Design review of the part built by this model. Coordinates are the model's own, in mm. A direction names the side the tool comes from. Give positions to 0.01 mm unless a question says otherwise; leave off trailing zeros. Order: outer loops, then holes, each group sorted by start corner. A loop starts at its lowest first (then second) coordinate and runs counter-clockwise, first axis right, second up. Notation, with made-up numbers: M 6.5,24.25 L 17.5,24.25 A12 ccw 17.5,35.25 Z; hole C 20,10.25 d11. An arc over 180 degrees is marked long. Answer as a JSON object with one key per item and string values.
from build123d import *

# Parameters (mm, degrees)
F0_W      = 31.8
F0_H      = 15.8
F1_DEPTH  = 4.8
F2_W      = 29.4
F2_H      = 13.4
F3_DEPTH  = 8.4
F4_R      = 2.409
F5_DEPTH  = 1.8
F6_R      = 1.3
F7_DEPTH  = 1.2
F8_R      = 2.409
F9_DEPTH  = 8.4
F10_W     = 0.3
F10_H     = 0.6
F11_DEPTH = 8.4
F12_W     = 0.6
F12_H     = 0.3
F13_DEPTH = 8.4
F14_W     = 0.8
F14_H     = 3.4696710694
F15_DEPTH = 6.4


with BuildPart() as f1:
    # F0 (on Top) → F1 (new body, symmetric)
    with BuildSketch(Plane.XY):
        Rectangle(F0_W, F0_H)
    extrude(amount=F1_DEPTH, both=True)

    # F2 (on face) → F3 (cut)
    with BuildSketch(Plane(origin=(0, 0, -4.8), x_dir=(1, 0, 0), z_dir=(0, 0, -1))):
        Rectangle(F2_W, F2_H)
    extrude(amount=-F3_DEPTH, mode=Mode.SUBTRACT)

    # F4 (on face) → F5 (join)
    with BuildSketch(Plane.XY.offset(4.8)):
        with Locations((-12.291, 4.2910612803)):
            Circle(F4_R)
        with Locations((12.291, 4.2910612803)):
            Circle(F4_R)
        with Locations((-12.291, -4.2910612803)):
            Circle(F4_R)
        with Locations((12.291, -4.2910612803)):
            Circle(F4_R)
        with Locations((-4.291, 4.2910612803)):
            Circle(F4_R)
        with Locations((4.291, 4.2910612803)):
            Circle(F4_R)
        with Locations((-4.291, -4.2910612803)):
            Circle(F4_R)
        with Locations((4.291, -4.2910612803)):
            Circle(F4_R)
    extrude(amount=F5_DEPTH)

    # F6 (on face) → F7 (cut)
    with BuildSketch(Plane(origin=(0, 0, 3.6), x_dir=(1, 0, 0), z_dir=(0, 0, -1))):
        with Locations((-11.8301756735, 4)):
            Circle(F6_R)
        with Locations((-3.8301756735, 5.6396185296)):
            Circle(F6_R)
        with Locations((4, 4)):
            Circle(F6_R)
        with Locations((12, 4)):
            Circle(F6_R)
        with Locations((-11.8301756735, -4)):
            Circle(F6_R)
        with Locations((-3.8301756735, -5.6396185296)):
            Circle(F6_R)
        with Locations((4, -4)):
            Circle(F6_R)
        with Locations((12, -4)):
            Circle(F6_R)
    extrude(amount=-F7_DEPTH, mode=Mode.SUBTRACT)

    # F8 (on face) → F9 (join, through all)
    with BuildSketch(Plane(origin=(0, 0, 3.6), x_dir=(1, 0, 0), z_dir=(0, 0, -1))):
        Circle(F8_R)
    extrude(amount=F9_DEPTH)

    # F10 (on face) → F11 (join, through all)
    with BuildSketch(Plane(origin=(0, 0, 3.6), x_dir=(1, 0, 0), z_dir=(0, 0, -1))):
        with Locations((-14.55, 4)):
            Rectangle(F10_W, F10_H)
        with Locations((-14.55, -4)):
            Rectangle(F10_W, F10_H)
        with Locations((14.55, 4)):
            Rectangle(F10_W, F10_H)
        with Locations((14.55, -4)):
            Rectangle(F10_W, F10_H)
    extrude(amount=F11_DEPTH)

    # F12 (on face) → F13 (join, through all)
    with BuildSketch(Plane(origin=(0, 0, 3.6), x_dir=(1, 0, 0), z_dir=(0, 0, -1))):
        with Locations((-11.8301756735, 6.55)):
            Rectangle(F12_W, F12_H)
        with Locations((-3.8301756735, 6.55)):
            Rectangle(F12_W, F12_H)
        with Locations((4, 6.55)):
            Rectangle(F12_W, F12_H)
        with Locations((12.3396486531, 6.55)):
            Rectangle(F12_W, F12_H)
        with Locations((-3.8301756735, -6.55)):
            Rectangle(F12_W, F12_H)
        with Locations((-11.8301756735, -6.55)):
            Rectangle(F12_W, F12_H)
        with Locations((4, -6.55)):
            Rectangle(F12_W, F12_H)
        with Locations((12.3396486531, -6.55)):
            Rectangle(F12_W, F12_H)
    extrude(amount=F13_DEPTH)

    # F14 (on face) → F15 (join)
    with BuildSketch(Plane(origin=(0, 0, 3.6), x_dir=(1, 0, 0), z_dir=(0, 0, -1))):
        with Locations((0, 4.9651644653)):
            Rectangle(F14_W, F14_H)
        with Locations((0, -4.9651644653)):
            Rectangle(F14_W, F14_H)
    extrude(amount=F15_DEPTH)


solid = f1.part
(1) We need section B-B (z = -0.5). Count the separate pieces of the cut face and the enclosed holes in it, plus the area to 3 significant figures.
Checked values:
{"separate pieces": "2", "enclosed holes": "1", "area": "134 mm^2"}
(2) We need section D-D (z = 5.25). Write out the cut boundary in (x, y), plus the area to 3 significant figures.
Checked values:
{"outline": "C -12.29,-4.29 d4.82; C -12.29,4.29 d4.82; C -4.29,-4.29 d4.82; C -4.29,4.29 d4.82; C 4.29,-4.29 d4.82; C 4.29,4.29 d4.82; C 12.29,-4.29 d4.82; C 12.29,4.29 d4.82", "area": "146 mm^2"}
(3) To check wall thickness, follow L1, parallel to X at y = 3.75, z = -1.75; L2, parallel to Y at x = 12, z = 4.55; L3, parallel to X at y = 4, z = 4.5. State the ranges of each line that lie inside material, in increasing order. Write a range as from..to.
Checked values:
{"L1": "x = -15.9..-14.4, -0.4..0.4, 14.4..15.9", "L2": "y = -7.9..-5.3, -2.7..2.7, 5.3..7.9", "L3": "x = -15.9..-13.13, -10.53..2.7, 5.3..10.7, 13.3..15.9"}
(4) We need section A-A (x = 7.5). Write out the cut boundary in (y, z).
Checked values:
{"outline": "M -7.9,-4.8 L -6.7,-4.8 L -6.7,3.6 L 6.7,3.6 L 6.7,-4.8 L 7.9,-4.8 L 7.9,4.8 L -7.9,4.8 Z"}
(5) We need section C-C (y = -1.5). Write out the cut boundary in (x, z), plus the area to 3 significant figures.
Checked values:
{"outline": "M -15.9,-4.8 L -14.7,-4.8 L -14.7,3.6 L -1.89,3.6 L -1.89,-4.8 L 1.89,-4.8 L 1.89,3.6 L 14.7,3.6 L 14.7,-4.8 L 15.9,-4.8 L 15.9,4.8 L -15.9,4.8 Z", "area": "90.0 mm^2"}
(6) Insertion check: pin 1 (6 mm diameter, centred on x = 7, y = -5, fed in from -Z); pin 2 (1.3 mm diameter, centred on x = 4.5, y = -4, fed in from -Z). Each pin has a flat end and moves straight along its axis. Give the tip position at first contact, or say it passes through.
Checked values:
{"pin 1": "stops at z = -4.8", "pin 2": "stops at z = 4.8"}
(7) Tool access review of faces 1 (the flat face through (-14.7, 0, -1)), 2 (the cylindrical face through (5.403, 2.154, 5.687)), 3 (the flat face through (0, -7.9, 0)): name each direction out of +Z, -Z, +X, -X, +Y, -Y from which nothing blocks a thin tool from reaching the whole face with its end or side.
Checked values:
{"face 1": "-Z", "face 2": "+Z", "face 3": "+Z, -Z, +X, -X, -Y"}
(8) Draft analysis for pull direction X (two halves, no side actions). For faces 4 (the flat face through (14.7, -5, -1)), 5 (the flat face through (-12, 4, 6.6)), state which applies: +X half, -X half, draft (parallel to the pull), parting line (faces both ways), or undercut.
Checked values:
{"face 4": "undercut", "face 5": "draft"}
